Source: CAD feature listing. Evaluate the final solid. Frame: model axes, mm. A direction names the side the tool comes from. Coordinates: 2 decimals unless noted, no trailing zeros. Loops run counter-clockwise (first coordinate to the right, second up) from the corner with the lowest first, then second, coordinate; pieces in that order, holes last. Notation, with made-up numbers: M -31.5,7.25 L -14.5,7.25 A21 ccw -14.5,45.25 Z; hole C 13.25,49 d8. An arc over 180 degrees is marked long. One line per question, with ' | ' between items. Start each with the question number.
1. Section query A-A, the plane z = -2.2. Output: boundary loops of the cut face in (x, y).
2. Mould query, pull axis X, two halves, no side actions, for faces 1 (the flat face through (0, -7.5, 0)), 2 (the cylindrical face through (0, 6, 0)), 3 (the flat face through (-2.5, 0, 0)). Classes: pulls with the +X half, pulls with the -X half, needs draft (parallel to the pull), parting line crosses it, or undercut.
3. Section query D-D, the plane z = -0.65. Output: boundary loops of the cut face in (x, y), and give its area (3 significant figures).
4. Pin query (flat end, axial travel): P1, Ø1.6, axis at x = 1, y = -7, coming from the +Z side; P2, Ø1.6, axis at x = 0.5, z = -2, coming from the -Y side. Return the tip coordinate at first contact, or that it passes through.
5. Section query C-C, the plane x = 0. Output: boundary loops of the cut face in (y, z).
6. Section query B-B, the plane y = 5. Output: boundary loops of the cut face in (x, z), and give its area (3 significant figures).
7. Ray query, probe 1 along Y at (x, z) = (0, 1.05); probe 2 along Y at (x, z) = (0, -0.55); probe 3 along Y at (x, z) = (1.55, 2). Return the intervals inside material, ascending.
8. Access query for faces 4 (the flat face through (0, -7, 1)), 5 (the flat face through (0, -3, 2)), 6 (the flat face through (0, 3, -2.5)), 7 (the flat face through (0, -1.5, -2)), 8 (the flat face through (0, -6, -2)). Directions: +Z, -Z, +X, -X, +Y, -Y. A direction counts if a zero-diameter tool reaches every point of the face in a straight line with its end or side. Return the directions, or none.
```python
from build123d import *

# Parameters (mm, degrees)
SKETCH2_W           = 5
SKETCH2_H           = 15
SKETCH2_R           = 1
BOSS_EXTRUDE1_DEPTH = 2.5
SKETCH3_W           = 1.5
SKETCH3_H           = 1.5
CUT_EXTRUDE1_DEPTH  = 10.354143467


with BuildPart() as part:
    # Sketch2 → Boss-Extrude1 (new, symmetric)
    with BuildSketch(Plane.XY):
        Rectangle(SKETCH2_W, SKETCH2_H)
        with Locations((0, 5)):
            Circle(SKETCH2_R, mode=Mode.SUBTRACT)
    extrude(amount=BOSS_EXTRUDE1_DEPTH, both=True)

    # Sketch3 → Cut-Extrude1 (cut, through all)
    with BuildSketch(Plane(origin=(2.5, 0, 0), x_dir=(0, 0, -1), z_dir=(1, 0, 0))):
        with Locations((-1.75, -2.25)):
            Rectangle(SKETCH3_W, SKETCH3_H)
        with Locations((-1.75, -6.75)):
            Rectangle(SKETCH3_W, SKETCH3_H)
        with Locations((1.75, -6.75)):
            Rectangle(SKETCH3_W, SKETCH3_H)
        with Locations((1.75, -2.25)):
            Rectangle(SKETCH3_W, SKETCH3_H)
    extrude(amount=-CUT_EXTRUDE1_DEPTH, mode=Mode.SUBTRACT)


solid = part.part
```
Taken from the geometry:
1) outline: M -2.5,-6 L 2.5,-6 L 2.5,-3 L -2.5,-3 Z; M -2.5,-1.5 L 2.5,-1.5 L 2.5,7.5 L -2.5,7.5 Z; hole C 0,5 d2
2) face 1: needs draft | face 2: undercut | face 3: pulls with the -X half
3) outline: M -2.5,-7.5 L 2.5,-7.5 L 2.5,7.5 L -2.5,7.5 Z; hole C 0,5 d2 | area: 71.9 mm^2
4) P1: z = 1 | P2: y = -6
5) outline: M -7.5,-1 L -6,-1 L -6,-2.5 L -3,-2.5 L -3,-1 L -1.5,-1 L -1.5,-2.5 L 4,-2.5 L 4,2.5 L -1.5,2.5 L -1.5,1 L -3,1 L -3,2.5 L -6,2.5 L -6,1 L -7.5,1 Z; M 6,-2.5 L 7.5,-2.5 L 7.5,2.5 L 6,2.5 Z
6) outline: M -2.5,-2.5 L -1,-2.5 L -1,2.5 L -2.5,2.5 Z; M 1,-2.5 L 2.5,-2.5 L 2.5,2.5 L 1,2.5 Z | area: 15.0 mm^2
7) probe 1: -6 to -3, -1.5 to 4, 6 to 7.5 | probe 2: -7.5 to 4, 6 to 7.5 | probe 3: -6 to -3, -1.5 to 7.5
8) face 4: +Z, +X, -X, -Y | face 5: +Z, +X, -X | face 6: -Z, +X, -X, +Y, -Y | face 7: -Z, +X, -X | face 8: -Z, +X, -X, -Y
